```python
from build123d import *

# Parameters (mm, degrees)
SKETCH1_R           = 4
SKETCH1_R_2         = 1.5
BOSS_EXTRUDE1_DEPTH = 8
SKETCH2_R           = 1.5
BOSS_EXTRUDE2_DEPTH = 5
SKETCH3_R           = 1.5
BOSS_EXTRUDE3_DEPTH = 6


with BuildPart() as part:
    # Sketch1 → Boss-Extrude1 (new body)
    with BuildSketch(Plane(origin=(0, 0, 0), x_dir=(1, 0, 0), z_dir=(0, 1, 0))):
        Circle(SKETCH1_R)
        Circle(SKETCH1_R_2, mode=Mode.SUBTRACT)
    extrude(amount=BOSS_EXTRUDE1_DEPTH)

    # Sketch2 → Boss-Extrude2 (add)
    with BuildSketch(Plane(origin=(0, 8, 0), x_dir=(1, 0, 0), z_dir=(0, 1, 0))):
        Circle(SKETCH2_R)
    extrude(amount=-BOSS_EXTRUDE2_DEPTH)

    # Sketch3 → Boss-Extrude3 (add)
    with BuildSketch(Plane(origin=(0, 8, 0), x_dir=(1, 0, 0), z_dir=(0, 1, 0))):
        Circle(SKETCH3_R)
    extrude(amount=BOSS_EXTRUDE3_DEPTH)


solid = part.part
```
The model under review builds one solid part; all positions refer to its coordinate system, in mm. A direction names the side the tool comes from. Give positions to 0.01 mm unless a question says otherwise; leave off trailing zeros. Loops run counter-clockwise (first coordinate to the right, second up) from the corner with the lowest first, then second, coordinate; pieces in that order, holes last. Notation, with made-up numbers: (8.25, 18.5) -> (13.25, 18.5) arc R27 cw to (13.25, 37.5) -> close; hole circle Ø9 at (12.25, 7). An arc over 180 degrees is marked (long way). Use CSV: the item, a comma, the result in double quotes.
1. To check wall thickness, follow probe 1 along Z at (x, y) = (0, 1.8); probe 2 along Y at (x, z) = (-1.5, 0.75). State the ranges of each line that lie inside material, in increasing order. Write a range as from..to.
Result:
probe 1,"z = -4..-1.5, 1.5..4"
probe 2,"y = 0..8"
2. Machinability: for faces 1 (the face through (0, 3, 0)), 2 (the face through (2, 0, 0)), 3 (the face through (-1.5, 10.96, -0.07)), which of the approach directions +Z, -Z, +X, -X, +Y, -Y give a long, thin tool a straight path to every point of the face, cutting with its end or side? Answer none if there is none.
Result:
face 1,"-Y"
face 2,"+Z, -Z, +X, -X, -Y"
face 3,"+Y"
3. For P1, Ø2, axis at y = 11.5, z = -0.5, coming from the -X side; P2, Ø1, axis at x = 2.5, y = 3.5, coming from the +Z side; P3, Ø1.5, axis at y = 9.5, z = -2, coming from the -X side, all flat-tipped, find the tip position at first contact; note any pin that passes through.
Result:
P1,"stops at x = -1.5"
P2,"stops at z = 3.46"
P3,"stops at x = -0.83"
4. Consider section C-C, the plane y = 5.25. Write out the cut boundary in (x, z), then the cut area to 3 significant figures.
Result:
outline,"circle Ø8 at (0, 0)"
area,"50.3 mm²"
5. The part is to be moulded in two halves that separate along X. For faces 4 (the face through (-1.5, 1.48, -0.07)), 5 (the face through (-0.867, 3.944, 3.905)), 6 (the face through (2, 8, 0)), say which applies: +X half, -X half, draft (parallel to the pull), parting line (faces both ways), or undercut.
Result:
face 4,"undercut"
face 5,"parting line"
face 6,"draft"
6. Consider section B-B, the plane x = 0. Write out the cut boundary in (y, z), then the cut area to 3 significant figures.
Result:
outline,"(0, -4) -> (8, -4) -> (8, -1.5) -> (14, -1.5) -> (14, 1.5) -> (8, 1.5) -> (8, 4) -> (0, 4) -> (0, 1.5) -> (3, 1.5) -> (3, -1.5) -> (0, -1.5) -> close"
area,"73.0 mm²"
7. Consider section D-D, the plane z = -2. Write out the cut boundary in (x, y).
Result:
outline,"(-3.46, 0) -> (3.46, 0) -> (3.46, 8) -> (-3.46, 8) -> close"
8. Consider section A-A, the plane z = 0. Write out the cut boundary in (x, y), then the cut area to 3 significant figures.
Result:
outline,"(-4, 0) -> (-1.5, 0) -> (-1.5, 3) -> (1.5, 3) -> (1.5, 0) -> (4, 0) -> (4, 8) -> (1.5, 8) -> (1.5, 14) -> (-1.5, 14) -> (-1.5, 8) -> (-4, 8) -> close"
area,"73.0 mm²"
